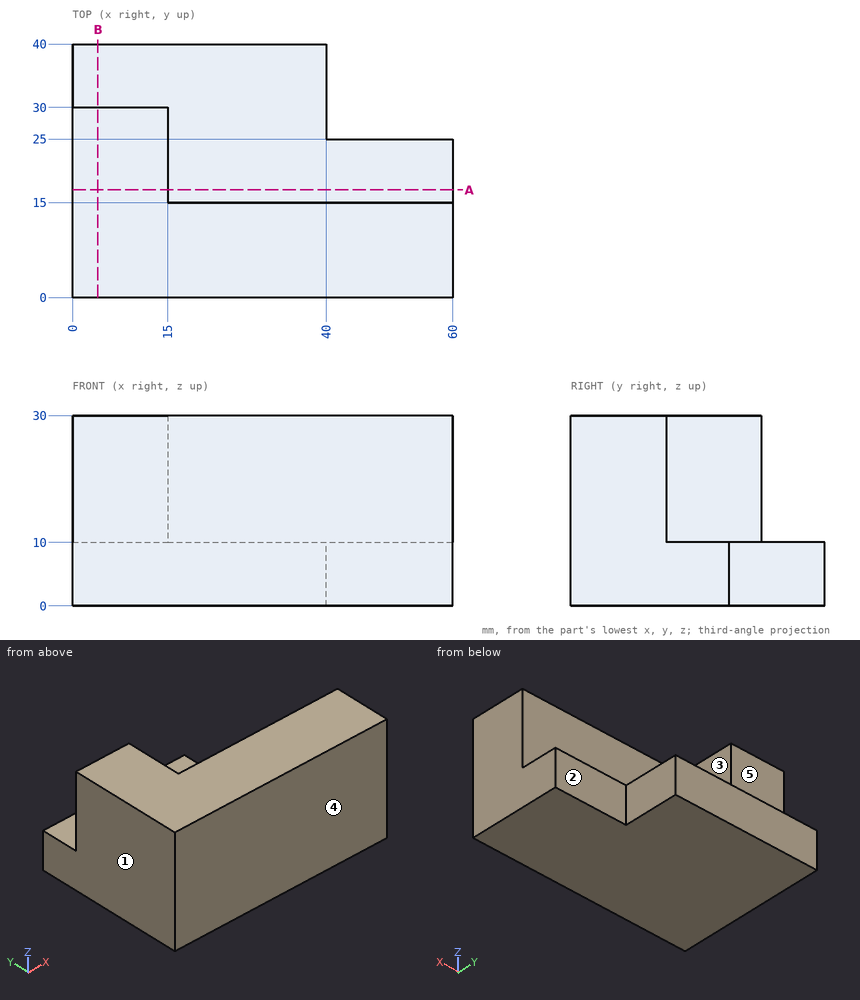
Geometry: see drawing. Coordinates: mm, zero at the bounding-box minimum. A direction names the side the tool comes from. Round coordinates to 2 decimals unless told otherwise and drop trailing zeros. Write each loop counter-clockwise with the first axis right and the second up, starting at its lowest first coordinate (ties: lowest second). Pieces come first, ordered by that corner, then holes.
Item 1: Pin query (flat end, axial travel): P1, Ø2, axis at x = 46, z = 7, coming from the +Y side; P2, Ø7.5, axis at x = 6, z = 17.5, coming from the +Y side; P3, Ø12.5, axis at x = 32, y = 30.5, coming from the +Z side; P4, Ø12, axis at x = 34.5, y = 11, coming from the -Z side. Return the tip coordinate at first contact, or that it passes through.
Item 2: Set-up query: the marked faces 1, 2, 3, 4 and 5. Return all of +Z, -Z, +X, -X, +Y, -Y with unobstructed straight access to the full face (end or side cutting, diameter ignored); none if empty.
Item 3: Section query A-A (y = 17). Return loops of the section in (x, z), plus the area to 3 significant figures.
Item 4: Material intervals for L1, parallel to Y at x = 17.5, z = 11.75; L2, parallel to Y at x = 9, z = 20.25, sorted ascending.
Item 5: Section query B-B (x = 4). Return loops of the section in (y, z), plus the area to 3 significant figures.
Completed:
1. P1: stops at y = 25
1. P2: stops at y = 30
1. P3: stops at z = 10
1. P4: stops at z = 0
2. face 1: +Z, -Z, -X, +Y, -Y
2. face 2: +Z, -Z, +X, +Y
2. face 3: +Z, +X, +Y
2. face 4: +Z, -Z, +X, -X, -Y
2. face 5: +Z, +X, -X, +Y
3. outline: (0, 0) - (60, 0) - (60, 10) - (15, 10) - (15, 30) - (0, 30) - close
3. area: 900 mm2
4. L1: y = 0 to 15
4. L2: y = 0 to 30
5. outline: (0, 0) - (40, 0) - (40, 10) - (30, 10) - (30, 30) - (0, 30) - close
5. area: 1,000 mm2
